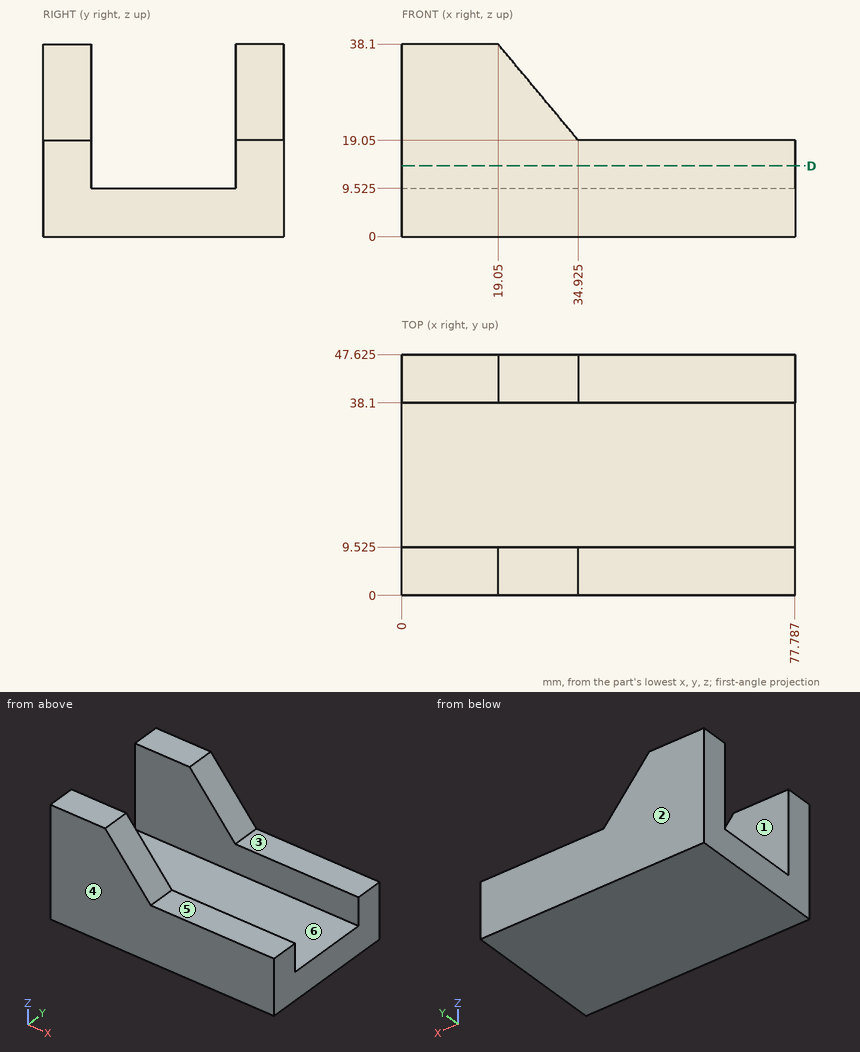
Design review of the part shown in the three views and the two pictorial views. Dimensions are in mm from the part's minimum x, y and z. A direction names the side the tool comes from. Coordinates: 2 decimals unless noted, no trailing zeros. Loops run counter-clockwise (first coordinate to the right, second up) from the corner with the lowest first, then second, coordinate; pieces in that order, holes last. Notation, with made-up numbers: M 8,-0.5 L 45,-0.5 A36 ccw 45,33.5 Z; hole C 28,-39 d7. An arc over 180 degrees is marked long. One line per question, with ' | ' between items.
(1) Wall thickness on probe 1 along Y at (x, z) = (7, 10) (1 decimal); probe 2 along Z at (x, y) = (8, 22.5) (1 decimal); probe 3 along Z at (x, y) = (44, 7): over which ranges is each line inside the solid? List them lowest first.
Filled in:
probe 1: y = 0 to 9.5, 38.1 to 47.6 | probe 2: z = 0 to 9.5 | probe 3: z = 0 to 19.05
(2) Draft analysis for pull direction Y (two halves, no side actions). For the marked faces 4, 5 and 6, state which applies: released by +Y, released by -Y, zero draft, split by the parting line, or undercut.
Filled in:
face 4: released by -Y | face 5: zero draft | face 6: undercut
(3) Machinability: for the marked faces 1, 2 and 3, which of the approach directions +Z, -Z, +X, -X, +Y, -Y give a long, thin tool a straight path to every point of the face, cutting with its end or side? Answer none if there is none.
Filled in:
face 1: +Z, +X, -X | face 2: +Z, -Z, +X, -X, +Y | face 3: +Z, +X, +Y, -Y
(4) For pin 1 Ø6 at (x, z) = (38.5, 23) entering from -Y; pin 2 Ø10.5 at (x, y) = (50, 6.5) entering from +Z; pin 3 Ø6 at (x, y) = (32, 41) entering from +Z, all flat-tipped, find the tip position at first contact; note any pin that passes through.
Filled in:
pin 1: passes through | pin 2: stops at z = 19.05 | pin 3: stops at z = 26.16
(5) We need section D-D (z = 14). Give the boundary of the cut face in (x, y) (1 decimal).
Filled in:
outline: M 0,0 L 77.8,0 L 77.8,9.5 L 0,9.5 Z; M 0,38.1 L 77.8,38.1 L 77.8,47.6 L 0,47.6 Z
